Part print with two shaded views. Sizes in mm from the minimum x, y, z corner. A direction names the side the tool comes from. Coordinates: 2 decimals unless noted, no trailing zeros. Order: outer loops, then holes, each group sorted by start corner. A loop starts at its lowest first (then second) coordinate and runs counter-clockwise, first axis right, second up. Notation, with made-up numbers: (-17.75, -5.5) - (14.25, -5.5) arc R26 cw to (14.25, 11.5) - close; hole circle Ø1 at (24.5, -38.75). An arc over 180 degrees is marked (long way). Return JSON: item names as keys, results as strings.
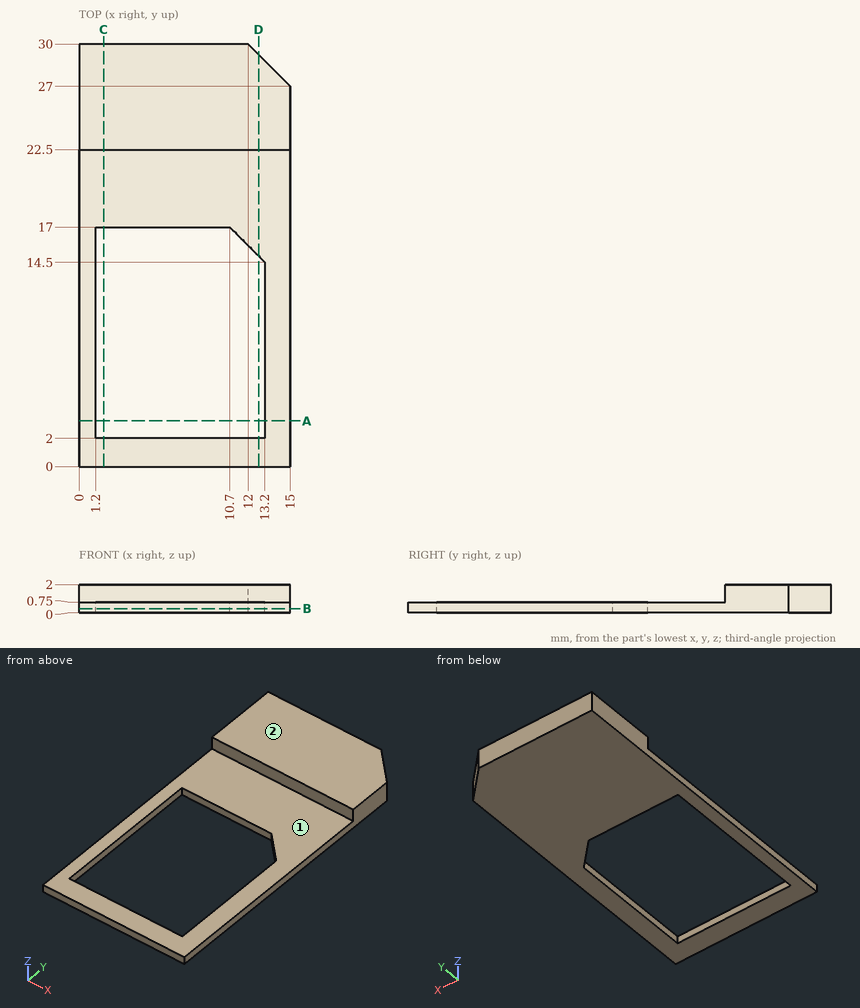
Item 1: Band-saw the part on C-C, the plane x = 1.75. List the corners of the cut face in (y, z), then the cut area to 3 significant figures.
Findings below:
{"outline": "(0, 0) - (2, 0) - (2, 0.75) - (0, 0.75) - close; (17, 0) - (30, 0) - (30, 2) - (22.5, 2) - (22.5, 0.75) - (17, 0.75) - close", "area": "20.6 mm²"}
Item 2: Band-saw the part on A-A, the plane y = 3.25. List the corners of the cut face in (x, z), then the cut area to 3 significant figures.
Findings below:
{"outline": "(0, 0) - (1.2, 0) - (1.2, 0.75) - (0, 0.75) - close; (13.2, 0) - (15, 0) - (15, 0.75) - (13.2, 0.75) - close", "area": "2.25 mm²"}
Item 3: Band-saw the part on B-B, the plane z = 0.3. List the corners of the cut face in (x, y).
Findings below:
{"outline": "(0, 0) - (15, 0) - (15, 27) - (12, 30) - (0, 30) - close; hole (1.2, 2) - (13.2, 2) - (13.2, 14.5) - (10.7, 17) - (1.2, 17) - close"}
Item 4: Wall check: L1, parallel to X at y = 9.5, z = 0.4; L2, parallel to Y at x = 9.5, z = 0.25; L3, parallel to Y at x = 1.5, z = 1.45. Give the ranges that are in metal, low to high. Write a range as [from, to].
Findings below:
{"L1": "x = [0, 1.2], [13.2, 15]", "L2": "y = [0, 2], [17, 30]", "L3": "y = [22.5, 30]"}
Item 5: Which spindle directions (+Z, -Z, +X, -X, +Y, -Y) get a long thin tool onto all of the face, cutting with end or side? Do the marked faces 1 and 2. Say none if no direction does.
Findings below:
{"face 1": "+Z, +X, -X, -Y", "face 2": "+Z, +X, -X, +Y, -Y"}
Item 6: Band-saw the part on D-D, the plane x = 12.75. List the corners of the cut face in (y, z).
Findings below:
{"outline": "(0, 0) - (2, 0) - (2, 0.75) - (0, 0.75) - close; (14.95, 0) - (29.25, 0) - (29.25, 2) - (22.5, 2) - (22.5, 0.75) - (14.95, 0.75) - close"}
Item 7: Drop flat-ended pins along their axis: P1, Ø8, axis at x = 5, y = 10, coming from the +Z side; P2, Ø1, axis at x = 9.5, z = 1, coming from the -Y side; P3, Ø1, axis at y = 5.5, z = 1.5, coming from the -X side. Give the stop position or say it passes through.
Findings below:
{"P1": "stops at z = 0.75", "P2": "stops at y = 0", "P3": "passes through"}
